Source: CAD feature listing. Evaluate the final solid. Frame: model axes, mm. A direction names the side the tool comes from. Round coordinates to 2 decimals unless told otherwise and drop trailing zeros. Loops run counter-clockwise (first coordinate to the right, second up) from the corner with the lowest first, then second, coordinate; pieces in that order, holes last. Notation, with made-up numbers: (-20, 65) - (12, 65) arc R17 cw to (12, 98) - close; hole circle Ø11 at (88.5, 26). An arc over 180 degrees is marked (long way). One line per question, with ' | ' between items.
from build123d import *

# Parameters (mm, degrees)
BOSS_EXTRUDE1_DEPTH = 3


with BuildPart() as part:
    # Sketch1 → Boss-Extrude1 (new body)
    with BuildSketch(Plane.XY.offset(-573)):
        Polygon((371.221, 43.742761671), (374.396, 43.742761671), (374.396, 51.45098076), (384.396, 51.45098076), (384.396, 16.438825445), (344.221, 16.438825445), (344.221, 31.443621916), (341.221, 31.443621916), (341.221, 16.438825445), (299.875, 16.438825445), (299.875, 31.443621916), (296.875, 31.443621916), (296.875, 16.438825445), (256.7, 16.438825445), (256.7, 43.443621916), (319.643036314, 43.443621916), (319.80460348, 35.648311515), (322.978935298, 35.713515129), (322.817368061, 43.508828946), (371.221, 51.450981405), align=None)
    extrude(amount=BOSS_EXTRUDE1_DEPTH)


solid = part.part
1. Section query B-B, the plane z = -571.5. Return loops of the section in (x, y) (3 decimals), plus the area to 3 significant figures.
Worked out:
outline: (256.7, 16.439) - (296.875, 16.439) - (296.875, 31.444) - (299.875, 31.444) - (299.875, 16.439) - (341.221, 16.439) - (341.221, 31.444) - (344.221, 31.444) - (344.221, 16.439) - (384.396, 16.439) - (384.396, 51.451) - (374.396, 51.451) - (374.396, 43.743) - (371.221, 43.743) - (371.221, 51.451) - (322.817, 43.509) - (322.979, 35.714) - (319.805, 35.648) - (319.643, 43.444) - (256.7, 43.444) - close | area: 3,610 mm2
2. Section query C-C, the plane x = 274.5. Return loops of the section in (y, z).
Worked out:
outline: (16.44, -573) - (43.44, -573) - (43.44, -570) - (16.44, -570) - close
3. Section query A-A, the plane y = 49.5. Return loops of the section in (x, z), plus the area to 3 significant figures.
Worked out:
outline: (359.33, -573) - (371.22, -573) - (371.22, -570) - (359.33, -570) - close; (374.4, -573) - (384.4, -573) - (384.4, -570) - (374.4, -570) - close | area: 65.7 mm2
4. Contact query for flat-ended pins moving along their axis: P1, Ø1.5, axis at y = 44, z = -571, coming from the -X side; P2, Ø1, axis at x = 297, z = -570.5, coming from the +Y side; P3, Ø1.5, axis at x = 342.5, z = -571, coming from the -Y side. Output: stop coordinate, or through.
Worked out:
P1: stops at x = 256.7 | P2: stops at y = 43.44 | P3: stops at y = 31.44
5. Material intervals for probe 1 along X at (y, z) = (27, -572.5) (3 decimals); probe 2 along Y at (x, z) = (318, -572.3); probe 3 along Y at (x, z) = (297.5, -570.05), sorted ascending.
Worked out:
probe 1: x = 256.7 to 296.875, 299.875 to 341.221, 344.221 to 384.396 | probe 2: y = 16.44 to 43.44 | probe 3: y = 31.44 to 43.44
6. Access query for faces 1 (the flat face through (379, 51.451, -572)), 2 (the flat face through (344.221, 24, -572)), 3 (the flat face through (321, 16.439, -572)), 4 (the flat face through (288, 43.444, -572)), 5 (the flat face through (373, 43.743, -572)). Directions: +Z, -Z, +X, -X, +Y, -Y. A direction counts if a zero-diameter tool reaches every point of the face in a straight line with its end or side. Return the directions, or none.
Worked out:
face 1: +Z, -Z, +X, -X, +Y | face 2: +Z, -Z, -Y | face 3: +Z, -Z, +X, -X, -Y | face 4: +Z, -Z, -X, +Y | face 5: +Z, -Z, +Y
7. Section query D-D, the plane y = 40.5. Return loops of the section in (x, z), plus the area to 3 significant figures.
Worked out:
outline: (256.7, -573) - (319.7, -573) - (319.7, -570) - (256.7, -570) - close; (322.88, -573) - (384.4, -573) - (384.4, -570) - (322.88, -570) - close | area: 374 mm2
8. Mould query, pull axis X, two halves, no side actions, for faces 6 (the flat face through (341.221, 24, -572)), 7 (the flat face through (384.396, 34, -572)), 8 (the flat face through (277, 16.439, -572)). Classes: released by +X, released by -X, zero draft, split by the parting line, or undercut.
Worked out:
face 6: undercut | face 7: released by +X | face 8: zero draft
